from build123d import *

# Parameters (mm, degrees)
F4_R     = 25
F4_R_2   = 22
F6_DEPTH = 150
F5_R     = 12
F5_R_2   = 10
F8_START = -12
F5_R_3   = 20
F8_DEPTH = 3


with BuildPart() as f6:
    # F4 (on Top) → F6 (new body, through all)
    with BuildSketch(Plane.XY):
        with Locations((0, -67.5)):
            Circle(F4_R)
        with Locations((0, -67.5)):
            Circle(F4_R_2, mode=Mode.SUBTRACT)
    extrude(amount=F6_DEPTH)

    # F5 (on offset) → F7 (join, up to the next surface of F6)
    with BuildSketch(Plane.XZ.offset(135)):
        with Locations((0, 125)):
            Circle(F5_R)
        with Locations((0, 125)):
            Circle(F5_R_2, mode=Mode.SUBTRACT)
        with Locations((0, 25)):
            Circle(F5_R)
        with Locations((0, 25)):
            Circle(F5_R_2, mode=Mode.SUBTRACT)
    extrude(until=Until.NEXT, dir=(0, 1, 0))

    # F5 (on offset) → F8 (join)
    with BuildSketch(Plane.XZ.offset(135).offset(F8_START)):
        with Locations((0, 125)):
            Circle(F5_R_3)
        with Locations((0, 125)):
            Circle(F5_R, mode=Mode.SUBTRACT)
        with Locations((0, 25)):
            Circle(F5_R_3)
        with Locations((0, 25)):
            Circle(F5_R, mode=Mode.SUBTRACT)
    extrude(amount=-F8_DEPTH)

    # F9: F6 across plane


with BuildPart() as f6_1:
    add(f6.part)
    add(f6.part.mirror(Plane.XZ.offset(67.5)))


solid = f6_1.part
Part model, mm, in its own coordinate system. A direction names the side the tool comes from. Coordinates: 2 decimals unless noted, no trailing zeros. Loops run counter-clockwise (first coordinate to the right, second up) from the corner with the lowest first, then second, coordinate; pieces in that order, holes last. Notation, with made-up numbers: (49.25, 5) - (96.25, 5) arc R22 cw to (96.25, 40) - close; hole circle Ø2 at (20, 50). An arc over 180 degrees is marked (long way). Write each question's results on one line, items separated by ' | '. Start each with the question number.
Q1. Slice it at D-D on y = -23. Give the cut face in (x, z).
Q2. Probe line 1 along Z through (x, y) = (0, -113); line 2 along X through (y, z) = (-34, 25); line 3 along Z through (x, y) = (-3, -39). List the from-to ranges inside material, lowest first.
Q3. Slice it at A-A on y = -67.5. Give the cut face in (x, z).
Q4. Which spindle directions (+Z, -Z, +X, -X, +Y, -Y) get a long thin tool onto all of the face, cutting with end or side? Do faces 3 (the cylindrical face through (-8.844, -129.084, 133.11)), 4 (the cylindrical face through (-11.99, -30.07, 25.53)), 5 (the cylindrical face through (-8.844, -5.916, 133.11)). Say none if no direction does.
Q5. Drop flat-ended pins along their axis: pin 1 Ø16 at (x, z) = (0, 125) entering from -Y; pin 2 Ø20 at (x, z) = (-2, 23) entering from -Y; pin 3 Ø5 at (y, z) = (-112, 117.5) entering from +X; pin 4 Ø5 at (x, y) = (-1.5, -22.5) entering from +Z. Give the stop position or say it passes through.
Q6. Two-plate mould, pull along Z, no slides. Class faces 1 (the flat face through (-5, -135, 34)), 2 (the flat face through (9, -120, 16)): +Z half, -Z half, draft (parallel to the pull), parting line (faces both ways), or undercut.
Q7. Slice it at C-C on x = -17. Give the cut face in (y, z), and give its area (3 significant figures).
Answer:
1) outline: circle Ø24 at (0, 25); circle Ø24 at (0, 125); hole circle Ø20 at (0, 25); hole circle Ø20 at (0, 125)
2) line 1: z = 13 to 15, 35 to 37, 113 to 115, 135 to 137 | line 2: x = -12 to -10, 10 to 12 | line 3: z = 13.38 to 15.46, 34.54 to 36.62, 113.38 to 115.46, 134.54 to 136.62
3) outline: (-25, 0) - (-22, 0) - (-22, 150) - (-25, 150) - close; (22, 0) - (25, 0) - (25, 150) - (22, 150) - close
4) face 3: -Y | face 4: none | face 5: +Y
5) pin 1: stops at y = -92.5 | pin 2: stops at y = -135 | pin 3: stops at x = 10.91 | pin 4: stops at z = 137
6) face 1: draft | face 2: undercut
7) outline: (-123, 14.46) - (-120, 14.46) - (-120, 35.54) - (-123, 35.54) - close; (-123, 114.46) - (-120, 114.46) - (-120, 135.54) - (-123, 135.54) - close; (-85.83, 0) - (-81.46, 0) - (-81.46, 150) - (-85.83, 150) - close; (-53.54, 0) - (-49.17, 0) - (-49.17, 150) - (-53.54, 150) - close; (-15, 14.46) - (-12, 14.46) - (-12, 35.54) - (-15, 35.54) - close; (-15, 114.46) - (-12, 114.46) - (-12, 135.54) - (-15, 135.54) - close | area: 1,560 mm2
